```python
from build123d import *

# Parameters (mm, degrees)
SKETCH1_W           = 8
SKETCH1_H           = 38
BOSS_EXTRUDE1_DEPTH = 2
SKETCH2_R           = 3.925
SKETCH2_R_2         = 2.925
BOSS_EXTRUDE2_DEPTH = 3
CUT_EXTRUDE1_START  = -3
SKETCH3_R           = 2.925
SKETCH3_R_2         = 0.5
CUT_EXTRUDE1_DEPTH  = 3
FILLET3_R           = 2


with BuildPart() as part:
    # Sketch1 → Boss-Extrude1 (new body)
    with BuildSketch(Plane(origin=(0, 0, 0), x_dir=(1, 0, 0), z_dir=(0, 1, 0))):
        with Locations((4, 19)):
            Rectangle(SKETCH1_W, SKETCH1_H)
    extrude(amount=BOSS_EXTRUDE1_DEPTH)

    # Sketch2 → Boss-Extrude2 (add)
    with BuildSketch(Plane.XZ):
        with Locations(Location((4, -19, 0), (0, 0, 270))):
            Circle(SKETCH2_R)
        with Locations(Location((4, -19, 0), (0, 0, 270))):
            Circle(SKETCH2_R_2, mode=Mode.SUBTRACT)
    extrude(amount=BOSS_EXTRUDE2_DEPTH)

    # Sketch3 → Cut-Extrude1 (cut)
    with BuildSketch(Plane.XZ.offset(CUT_EXTRUDE1_START)):
        with Locations(Location((4, -19, 0), (0, 0, 270))):
            Circle(SKETCH3_R)
        with Locations(Location((4, -4, 0), (0, 0, 270))):
            Circle(SKETCH3_R_2)
        with Locations(Location((4, -8, 0), (0, 0, 270))):
            Circle(SKETCH3_R_2)
        with Locations(Location((4, -12, 0), (0, 0, 270))):
            Circle(SKETCH3_R_2)
        with Locations(Location((4, -26, 0), (0, 0, 270))):
            Circle(SKETCH3_R_2)
        with Locations(Location((4, -30, 0), (0, 0, 270))):
            Circle(SKETCH3_R_2)
        with Locations(Location((4, -34, 0), (0, 0, 270))):
            Circle(SKETCH3_R_2)
    extrude(amount=CUT_EXTRUDE1_DEPTH, mode=Mode.SUBTRACT)

    # Fillet3
    fillet3_edges = [part.edges().sort_by_distance(p)[0] for p in [
        (0, 1, -38),
        (8, 1, -38),
        (8, 1, 0),
        (0, 1, 0),
    ]]
    fillet(fillet3_edges, radius=FILLET3_R)


solid = part.part
```
The model under review builds one solid part; all positions refer to its coordinate system, in mm. A direction names the side the tool comes from. Give positions to 0.01 mm unless a question says otherwise; leave off trailing zeros. Write each loop counter-clockwise with the first axis right and the second up, starting at its lowest first coordinate (ties: lowest second). Pieces come first, ordered by that corner, then holes. Notation, with made-up numbers: (21, 85.25) - (80, 85.25) arc R19 cw to (80, 96.25) - close; hole circle Ø3 at (30, 55). An arc over 180 degrees is marked (long way). Answer in a Markdown table with one row per item. Add a question column.
1. Wall thickness on line 1 along X through (y, z) = (1.2, -8); line 2 along X through (y, z) = (0.25, -19) (3 decimals); line 3 along Y through (x, z) = (5.5, -2): over which ranges is each line inside the solid? List them lowest first. Write a range as [from, to].
2. Tool access review of faces 5 (the cylindrical face through (0.57, 1.01, -37.4)), 6 (the cylindrical face through (4.17, -1.48, -15.08)): name each direction out of +Z, -Z, +X, -X, +Y, -Y from which nothing blocks a thin tool from reaching the whole face with its end or side.
3. We need section C-C on x = 5.5. Write out the cut boundary in (y, z), then the cut area to 3 significant figures.
4. We need section D-D on y = -1.55. Write out the cut boundary in (x, z) (3 decimals), then the cut area to 3 significant figures.
5. Insertion check: P1, Ø3, axis at y = -2, z = -5.5, coming from the +X side; P2, Ø2.5, axis at x = 5, z = -10.5, coming from the -Y side. Each pin has a flat end and moves straight along its axis. Give the tip position at first contact, or say it passes through.
6. We need section B-B on y = 0.95. Write out the cut boundary in (x, z) (3 decimals), then the cut area to 3 significant figures.
7. Draft analysis for pull direction X (two halves, no side actions). For faces 1 (the flat face through (8, 1, -19)), 2 (the cylindrical face through (0.57, 1.01, -0.6)), 3 (the cylindrical face through (4, 1, -33.5)), 4 (the flat face through (4, 1, 0)), state which applies: +X half, -X half, draft (parallel to the pull), parting line (faces both ways), or undercut.
8. We need section A-A on z = -12. Write out the cut boundary in (x, y), then the cut area to 3 significant figures.
Ans:
| question | item | result |
|---|---|---|
| 1 | line 1 | x = [0, 3.5], [4.5, 8] |
| 1 | line 2 | x = [0, 1.075], [6.925, 8] |
| 1 | line 3 | y = [0, 2] |
| 2 | face 5 | -Z, -X, +Y, -Y |
| 2 | face 6 | -Y |
| 3 | outline | (-3, -22.63) - (0, -22.63) - (0, -38) - (2, -38) - (2, -21.51) - (-3, -21.51) - close; (-3, -16.49) - (2, -16.49) - (2, 0) - (0, 0) - (0, -15.37) - (-3, -15.37) - close |
| 3 | area | 72.7 mm^2 |
| 4 | outline | circle Ø7.85 at (4, -19); hole circle Ø5.85 at (4, -19) |
| 4 | area | 21.5 mm^2 |
| 5 | P1 | passes through |
| 5 | P2 | stops at y = 0 |
| 6 | outline | (0, -36) arc R2 ccw to (2, -38) - (6, -38) arc R2 ccw to (8, -36) - (8, -2) arc R2 ccw to (6, 0) - (2, 0) arc R2 ccw to (0, -2) - close; hole circle Ø5.85 at (4, -19); hole circle Ø1 at (4, -34); hole circle Ø1 at (4, -30); hole circle Ø1 at (4, -26); hole circle Ø1 at (4, -12); hole circle Ø1 at (4, -8); hole circle Ø1 at (4, -4) |
| 6 | area | 269 mm^2 |
| 7 | face 1 | +X half |
| 7 | face 2 | -X half |
| 7 | face 3 | undercut |
| 7 | face 4 | draft |
| 8 | outline | (0, 0) - (3.5, 0) - (3.5, 2) - (0, 2) - close; (4.5, 0) - (8, 0) - (8, 2) - (4.5, 2) - close |
| 8 | area | 14.0 mm^2 |
